Autodesk Inventor part; units mm, degrees
ref_plane "Work Plane1" through (40, 0, 60) normal (0, 0, -1) x (0, -1, 0)
ref_plane "YZ Plane" through (0, 0, 0) normal (1, 0, 0) x (0, 1, 0)
ref_plane "XZ Plane" through (0, 0, 0) normal (0, 1, 0) x (-1, 0, 0)
sketch "Sketch1" plane through (0, 0, 0) normal (0, 1, 0) x (-1, 0, 0)
  arc A0 (26.4575, 30) -> (-26.4575, 30) centre (0, 0) ccw construction
  arc A1 (40, 60) -> (-40, 60) centre (0, 60) ccw
  line L0 (0, 100) -> (0, 0) construction
  line L1 (40, 60) -> (40, 0)
  line L2 (-40, 60) -> (-40, 0)
  arc A2 (26.4575, 30) -> (40, 60) centre (0, 60) ccw construction
  arc A3 (40, 0) -> (26.4575, 30) centre (0, 0) ccw construction
  arc A4 (-40, 60) -> (26.4575, 30) centre (0, 60) ccw construction
  arc A5 (-26.4575, 30) -> (-40, 0) centre (0, 0) ccw construction
  arc A6 (-40, 0) -> (40, 0) centre (0, 0) ccw
  circle A7 centre (0, 0) radius 5
  dimension "d0" = 80
  dimension "d1" = 80
  dimension "d2" = 100
  dimension "d3" = 10
extrude "Extrusion1" add sketch "Sketch1" along normal mid plane 90
sketch "Sketch2" plane through (0, 0, 0) normal (0, 1, 0) x (-1, 0, 0)
  circle A0 centre (0, 0) radius 5
  circle A1 centre (0, 0) radius 45
  dimension "d6" = 90
extrude "Extrusion2" cut sketch "Sketch2" along normal mid plane 70
fillet "Fillet1" radius 2 10 edges at (40, 0, 20.6155) (-40, 0, 20.6155) (0, 45, -40) (-40, 45, 30) (0, 45, 100) (40, 45, 30) (0, -45, 100) (-40, -45, 30) (0, -45, -40) (40, -45, 30)
ref_plane "Work Plane1" through (40, 0, 60) normal (0, 0, -1) x (0, -1, 0)
sketch "Sketch3" plane through (40, 0, 60) normal (0, 0, -1) x (0, -1, 0)
  circle A0 centre (-13.55, 40) radius 30
  line L0 (0, 40) -> (-13.55, 40)
  dimension "d10" = 60
  dimension "d11" = 13.55
extrude "Extrusion3" add sketch "Sketch3" against normal blind 50
sketch "Sketch4" plane through (0, 13.55, 110) normal (0, 0, 1) x (1, 0, 0)
  circle A0 centre (0, 0) radius 30
  circle A1 centre (0, 0) radius 25
  point P0 (0, -13.55)
  dimension "d14" = 50
extrude "Extrusion4" cut sketch "Sketch4" against normal blind 10 contours A1
fillet "Fillet2" radius 2 2 edges at (0, 43.55, 110) (-25, 13.55, 110)
properties part number "Wirst2"
The listing builds one solid part. Answer for the finished solid, in the listing's coordinates (mm). A direction names the side the tool comes from. Round coordinates to 2 decimals unless told otherwise and drop trailing zeros. Write each loop counter-clockwise with the first axis right and the second up, starting at its lowest first coordinate (ties: lowest second). Pieces come first, ordered by that corner, then holes. Notation, with made-up numbers: M 33.25,58 L 51.25,58 A14 cw 51.25,65 Z; hole C 48,-24.5 d4. An arc over 180 degrees is marked long. Write each question's results on one line, items separated by ' | '. Start each with the question number.
(1) The part is cut by section B-B, the plane x = 0. Give the number of separate pieces and of enclosed holes in the cut face, and give its area (3 significant figures).
(2) For faces 1 (the cylindrical face through (-0.88, -39.06, -39.99)), 2 (the flat face through (0, 14, 100)), 3 (the cylindrical face through (38.585, -0.49, 25.746)), determine the directions among +Z, -Z, +X, -X, +Y, -Y from which every point of the face is accessible in a straight line to the end or side of a thin tool.
(3) Find the intervals of material crossed by line 1 (Z direction, x = 0, y = -43); line 2 (Y direction, x = 3.5, z = 18.5); line 3 (Y direction, x = 0, z = 106), in increasing order.
(4) The part is cut by section C-C, the plane y = 13.55. Write down the section's boundary in (x, z).
(5) This flat-tipped pin is pushed along its axis until it touches: P1, Ø1.5, axis at x = 2, y = -9.5, coming from the +Z side. Where does it stop, or does it pass through?
(6) The part is cut by section A-A, the plane z = 15. Write down the section's boundary in (x, y), and give its area (3 significant figures).
(7) Determine the mould class of faces 4 (the flat face through (-8, 35, 3)), 5 (the flat face through (1, 45, 31)), 6 (the cylindrical face through (0.88, -19.71, 99.99)) for opening direction X: +X half, -X half, draft (parallel to the pull), parting line (faces both ways), or undercut.
Worked answers:
1) separate pieces: 3 | enclosed holes: 0 | area: 6,540 mm²
2) face 1: -Z, +Y, -Y | face 2: +Z | face 3: -Z
3) line 1: z = -40 to -5, 5 to 100 | line 2: y = -45 to -35, 35 to 45 | line 3: y = -16.45 to -11.45, 38.55 to 43.55
4) outline: M -40,27.66 A2 ccw -36.38,26.48 A45 cw 36.38,26.48 A2 ccw 40,27.66 L 40,60 A40 ccw 30,86.46 L 30,108 A2 ccw 28,110 L 27,110 A2 ccw 25,108 L 25,100 L -25,100 L -25,108 A2 ccw -27,110 L -28,110 A2 ccw -30,108 L -30,86.46 A40 ccw -40,60 Z
5) P1: stops at z = 100
6) outline: M -40,-43 A2 ccw -38,-45 L 38,-45 A2 ccw 40,-43 L 40,-35 L -40,-35 Z; M -40,35 L 40,35 L 40,43 A2 ccw 38,45 L -38,45 A2 ccw -40,43 Z | area: 1,600 mm²
7) face 4: undercut | face 5: draft | face 6: parting line
